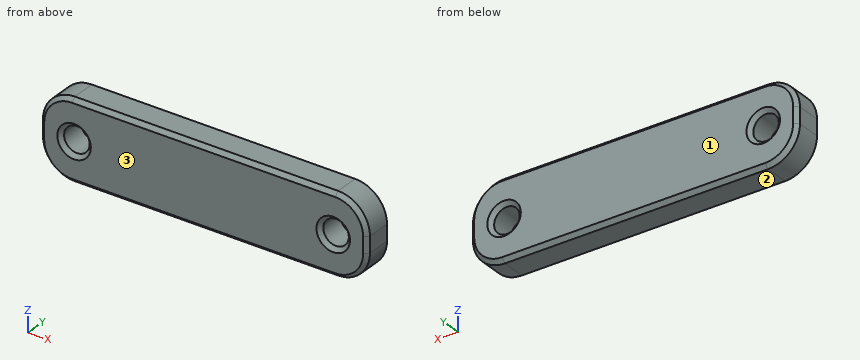
```python
from build123d import *

# Parameters (mm, degrees)
SKETCH1_W           = 41
SKETCH1_H           = 10
SKETCH1_R           = 1.6
BOSS_EXTRUDE1_DEPTH = 4
FILLET1_R           = 4
CHAMFER1_SIZE       = 0.5


with BuildPart() as part:
    # Sketch1 → Boss-Extrude1 (new body)
    with BuildSketch(Plane(origin=(0, 0, 0), x_dir=(1, 0, 0), z_dir=(0, 1, 0))):
        Rectangle(SKETCH1_W, SKETCH1_H)
        with Locations(Location((-16.25, 0, 0), (0, 0, 270))):
            Circle(SKETCH1_R, mode=Mode.SUBTRACT)
        with Locations(Location((16.25, 0, 0), (0, 0, 270))):
            Circle(SKETCH1_R, mode=Mode.SUBTRACT)
    extrude(amount=BOSS_EXTRUDE1_DEPTH)

    # Fillet1
    fillet1_edges = [part.edges().sort_by_distance(p)[0] for p in [
        (20.5, 2, 5),
        (-20.5, 2, 5),
        (-20.5, 2, -5),
        (20.5, 2, -5),
    ]]
    fillet(fillet1_edges, radius=FILLET1_R)

    # Chamfer1
    chamfer1_edges = [part.edges().sort_by_distance(p)[0] for p in [
        (-16.25, 0, -1.6),
        (-16.25, 4, -1.6),
        (16.25, 0, -1.6),
        (16.25, 4, -1.6),
        (0, 0, -5),
        (0, 4, -5),
        (20.5, 0, 0),
        (0, 0, 5),
        (-20.5, 0, 0),
        (-19.328427125, 0, -3.828427125),
        (-19.328427125, 0, 3.828427125),
        (19.328427125, 0, 3.828427125),
        (19.328427125, 0, -3.828427125),
        (20.5, 4, 0),
        (-20.5, 4, 0),
        (0, 4, 5),
        (-19.328427125, 4, -3.828427125),
        (-19.328427125, 4, 3.828427125),
        (19.328427125, 4, 3.828427125),
        (19.328427125, 4, -3.828427125),
    ]]
    chamfer(chamfer1_edges, length=CHAMFER1_SIZE)


solid = part.part
```
CAD build for the part. Positions are in the model's coordinates, mm. Face numbers are marked on the shaded views. Give positions to 0.01 mm unless a question says otherwise; leave off trailing zeros. Loops run counter-clockwise (first coordinate to the right, second up) from the corner with the lowest first, then second, coordinate; pieces in that order, holes last. Notation, with made-up numbers: (20.5, 33) -> (53.5, 33) arc R17 cw to (53.5, 41) -> close; hole circle Ø3 at (-35.75, 23). An arc over 180 degrees is marked (long way). Use a Markdown table: item, result.
1. Flat gauge pin, fed straight in: pin 1 (3.5 mm diameter, centred on x = -16.25, z = 0, fed in from +Y). Where does the tip first touch, or does it go through?
Check result:
| item | result |
|---|---|
| pin 1 | stops at y = 3.65 |
2. Slice it at B-B (y = 2.65). List the corners of the cut face in (x, z), plus the area to 3 significant figures.
Check result:
| item | result |
|---|---|
| outline | (-20.5, -1) arc R4 ccw to (-16.5, -5) -> (16.5, -5) arc R4 ccw to (20.5, -1) -> (20.5, 1) arc R4 ccw to (16.5, 5) -> (-16.5, 5) arc R4 ccw to (-20.5, 1) -> close; hole circle Ø3.2 at (-16.25, 0); hole circle Ø3.2 at (16.25, 0) |
| area | 380 mm^2 |
3. Wall check: L1, parallel to X at y = 2.5, z = 0; L2, parallel to X at y = 3.35, z = 0.75; L3, parallel to Z at x = 15.5, y = 1.55. Give the ranges that are in metal, low to high. Write a range as [from, to].
Check result:
| item | result |
|---|---|
| L1 | x = [-20.5, -17.85], [-14.65, 14.65], [17.85, 20.5] |
| L2 | x = [-20.5, -17.66], [-14.84, 14.84], [17.66, 20.5] |
| L3 | z = [-5, -1.41], [1.41, 5] |
4. Mould opens along Y. For the marked faces 1, 2 and 3 say: pulls with the +Y half, pulls with the -Y half, needs draft (parallel to the pull), parting line crosses it, or undercut.
Check result:
| item | result |
|---|---|
| face 1 | pulls with the +Y half |
| face 2 | needs draft |
| face 3 | pulls with the -Y half |
5. Slice it at A-A (z = 0). List the corners of the cut face in (x, y).
Check result:
| item | result |
|---|---|
| outline | (-20.5, 0.5) -> (-20, 0) -> (-18.35, 0) -> (-17.85, 0.5) -> (-17.85, 3.5) -> (-18.35, 4) -> (-20, 4) -> (-20.5, 3.5) -> close; (-14.65, 0.5) -> (-14.15, 0) -> (14.15, 0) -> (14.65, 0.5) -> (14.65, 3.5) -> (14.15, 4) -> (-14.15, 4) -> (-14.65, 3.5) -> close; (17.85, 0.5) -> (18.35, 0) -> (20, 0) -> (20.5, 0.5) -> (20.5, 3.5) -> (20, 4) -> (18.35, 4) -> (17.85, 3.5) -> close |
